from build123d import *

# Parameters (mm, degrees)
BOSS_EXTRUDE1_DEPTH = 150
SKETCH4_R           = 1.65
CUT_EXTRUDE1_DEPTH  = 7


with BuildPart() as part:
    # Sketch1 → Boss-Extrude1 (new body)
    with BuildSketch(Plane.XY):
        Polygon((-75.5, 3.5), (75.5, 3.5), (75.5, -3.5), (23.2, -3.5), (23.2, -13.5), (17.2, -13.5), (17.2, -3.5), (-17.2, -3.5), (-17.2, -13.5), (-23.2, -13.5), (-23.2, -3.5), (-75.5, -3.5), align=None)
    extrude(amount=BOSS_EXTRUDE1_DEPTH)

    # Sketch4 → Cut-Extrude1 (cut)
    with BuildSketch(Plane.XZ.offset(3.5)):
        with Locations((-10, 6)):
            Circle(SKETCH4_R)
        with Locations((10, 6)):
            Circle(SKETCH4_R)
        with Locations((-10, 144)):
            Circle(SKETCH4_R)
        with Locations((10, 144)):
            Circle(SKETCH4_R)
    extrude(amount=-CUT_EXTRUDE1_DEPTH, mode=Mode.SUBTRACT)


solid = part.part
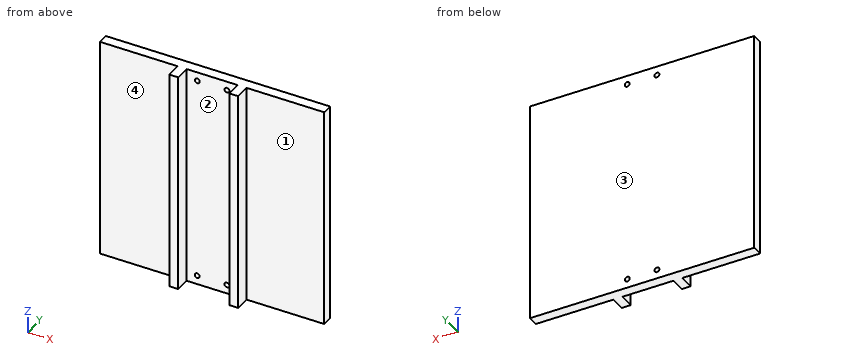
Verification items for the finished model (mm, model axes). Face numbers are marked on the shaded views. A direction names the side the tool comes from. Give positions to 0.01 mm unless a question says otherwise; leave off trailing zeros. Write each loop counter-clockwise with the first axis right and the second up, starting at its lowest first coordinate (ties: lowest second). Pieces come first, ordered by that corner, then holes. Notation, with made-up numbers: M 64.25,65 L 93.25,65 A6 cw 93.25,72 Z; hole C 85,69 d2. An arc over 180 degrees is marked long. Put each result on its own line as item: value. Start each with the question number.
1. Set-up check for the marked faces 3 and 4: record each of +Z, -Z, +X, -X, +Y, -Y from which the full face is reachable in a straight line by a thin tool's end or side.
2. Section check B-B (z = 80). Record the cut outline in (x, y), and give its area (3 significant figures).
3. Scan lines: line 1 along Z through (x, y) = (-10, 2); line 2 along X through (y, z) = (0, 144); line 3 along X through (y, z) = (-4.5, 137.5). Record each from-to range of solid material in increasing order. Write a range as [from, to].
4. Go/stop test with flat-tipped pins: pin 1 Ø6 at (x, z) = (-53, 55) entering from -Y; pin 2 Ø8 at (y, z) = (-10.5, 80) entering from -X. Record where each tip stops, or that it passes through.
5. Section check A-A (y = -5.25). Record the cut outline in (x, z).
6. Draft check along X on the marked faces 1 and 2. Enter one of: +X half, -X half, draft (parallel to the pull), parting line (faces both ways), or undercut.
7. Section check C-C (x = 15). Record the cut outline in (y, z).
Answer list:
1. face 3: +Z, -Z, +X, -X, +Y
1. face 4: +Z, -Z, -X, -Y
2. outline: M -75.5,-3.5 L -23.2,-3.5 L -23.2,-13.5 L -17.2,-13.5 L -17.2,-3.5 L 17.2,-3.5 L 17.2,-13.5 L 23.2,-13.5 L 23.2,-3.5 L 75.5,-3.5 L 75.5,3.5 L -75.5,3.5 Z
2. area: 1,180 mm2
3. line 1: [0, 4.35], [7.65, 142.35], [145.65, 150]
3. line 2: [-75.5, -11.65], [-8.35, 8.35], [11.65, 75.5]
3. line 3: [-23.2, -17.2], [17.2, 23.2]
4. pin 1: y = -3.5
4. pin 2: x = -23.2
5. outline: M -23.2,0 L -17.2,0 L -17.2,150 L -23.2,150 Z; M 17.2,0 L 23.2,0 L 23.2,150 L 17.2,150 Z
6. face 1: draft
6. face 2: undercut
7. outline: M -3.5,0 L 3.5,0 L 3.5,150 L -3.5,150 Z
